```python
from build123d import *

# Parameters (mm, degrees)
F0_W      = 149
F0_H      = 43
F1_DEPTH  = 7
F2_T      = -1.6
F3_DEPTH  = 1
F4_W      = 1.6
F4_H      = 5
F5_DEPTH  = 6.6
F6_W      = 5
F6_H      = 1.0360542744
F7_DEPTH  = 1
F8_SIZE   = 1
F9_W      = 5
F9_H      = 1.0135311693
F10_DEPTH = 1
F11_SIZE  = 1
F12_W     = 6.7361369729
F12_H     = 9.1
F13_DEPTH = 25


with BuildPart() as f1:
    # F0 (on Top) → F1 (new body)
    with BuildSketch(Plane.XY):
        with Locations((74.5, -21.5)):
            Rectangle(F0_W, F0_H)
    extrude(amount=F1_DEPTH)

    # F2
    f2_openings = [f1.faces().sort_by_distance(p)[0] for p in [
        (74.5, -21.5, 7),
    ]]
    offset(amount=F2_T, openings=f2_openings)

    # F3 (add): a face of the model
    f3_faces = [f1.faces().sort_by_distance(p)[0] for p in [
        (74.5, -21.5, 1.6),
    ]]
    extrude(f3_faces, amount=F3_DEPTH)

    # F4 (on face) → F5 (join)
    with BuildSketch(Plane.XY.offset(7)):
        with Locations((0.8, -6.7)):
            Rectangle(F4_W, F4_H)
        with Locations((0.8, -36.3)):
            Rectangle(F4_W, F4_H)
        with Locations((148.2, -6.7)):
            Rectangle(F4_W, F4_H)
        with Locations((148.2, -36.3)):
            Rectangle(F4_W, F4_H)
    extrude(amount=F5_DEPTH)

    # F6 (on face) → F7 (join)
    with BuildSketch(Plane(origin=(0, 0, 0), x_dir=(0, -1, 0), z_dir=(-1, 0, 0))):
        with Locations((6.7, 13.0819728628)):
            Rectangle(F6_W, F6_H)
        with Locations((36.3, 13.0819728628)):
            Rectangle(F6_W, F6_H)
    extrude(amount=F7_DEPTH)

    # F8
    f8_edges = [f1.edges().sort_by_distance(p)[0] for p in [
        (-1, -6.7, 13.6),
        (-1, -36.3, 13.6),
    ]]
    chamfer(f8_edges, length=F8_SIZE)

    # F9 (on face) → F10 (join)
    with BuildSketch(Plane.YZ.offset(149)):
        with Locations((-36.3, 13.0932344154)):
            Rectangle(F9_W, F9_H)
        with Locations((-6.7, 13.0932344154)):
            Rectangle(F9_W, F9_H)
    extrude(amount=F10_DEPTH)

    # F11
    f11_edges = [f1.edges().sort_by_distance(p)[0] for p in [
        (150, -36.3, 13.6),
        (150, -6.7, 13.6),
    ]]
    chamfer(f11_edges, length=F11_SIZE)

    # F12 (on face) → F13 (cut)
    with BuildSketch(Plane(origin=(0, 0, 0), x_dir=(1, 0, 0), z_dir=(0, 0, -1))):
        with Locations((77.8680684865, 26.05)):
            Rectangle(F12_W, F12_H)
        with Locations((71.1319315135, 26.05)):
            Rectangle(F12_W, F12_H)
        with Locations((77.8680684865, 16.95)):
            Rectangle(F12_W, F12_H)
        with Locations((71.1319315135, 16.95)):
            Rectangle(F12_W, F12_H)
    extrude(amount=-F13_DEPTH, mode=Mode.SUBTRACT)


solid = f1.part
```
CAD build for the part. Positions are in the model's coordinates, mm. A direction names the side the tool comes from. Round coordinates to 2 decimals unless told otherwise and drop trailing zeros. Write each loop counter-clockwise with the first axis right and the second up, starting at its lowest first coordinate (ties: lowest second). Pieces come first, ordered by that corner, then holes. Notation, with made-up numbers: M -27,-15.75 L 6,-15.75 A13 ccw 6,-7.75 Z; hole C -14,74 d10. An arc over 180 degrees is marked long. One line per question, with ' | ' between items.
1. Cut at C-C on y = -18. Write the cut outline in (x, z).
Working result:
outline: M 0,0 L 67.76,0 L 67.76,2.6 L 1.6,2.6 L 1.6,7 L 0,7 Z; M 81.24,0 L 149,0 L 149,7 L 147.4,7 L 147.4,2.6 L 81.24,2.6 Z
2. Probe L1, parallel to X at y = -30.5, z = 4; L2, parallel to Y at x = 45, z = 4.5; L3, parallel to X at y = -15, z = 2.5. List the from-to ranges inside material, lowest first. Write a range as from..to.
Working result:
L1: 0..1.6, 147.4..149 | L2: -43..-41.4, -1.6..0 | L3: 0..67.76, 81.24..149
3. Which spindle directions (+Z, -Z, +X, -X, +Y, -Y) get a long thin tool onto all of the face, cutting with end or side? Do faces 1 (the flat face through (73, -1.6, 5)), 2 (the flat face through (1, -4.2, 10)), 3 (the flat face through (74, -12.4, 1)). Say none if no direction does.
Working result:
face 1: +Z | face 2: +Z, +X, -X, +Y | face 3: +Z, -Z
4. Cut at A-A on x = 69.5. Write the cut outline in (y, z), and give its area (3 significant figures).
Working result:
outline: M -43,0 L -30.6,0 L -30.6,2.6 L -41.4,2.6 L -41.4,7 L -43,7 Z; M -12.4,0 L 0,0 L 0,7 L -1.6,7 L -1.6,2.6 L -12.4,2.6 Z | area: 78.6 mm2
5. Cut at B-B on z = 5.25. Write the cut outline in (x, y).
Working result:
outline: M 0,-43 L 149,-43 L 149,0 L 0,0 Z; hole M 1.6,-41.4 L 147.4,-41.4 L 147.4,-1.6 L 1.6,-1.6 Z
6. Pin check, flat tips, straight feed: pin 1 Ø1.8 at (x, y) = (0.5, -18) entering from +Z; pin 2 Ø3.5 at (y, z) = (-13.5, 5.5) entering from +X; pin 3 Ø1.3 at (x, z) = (149, 9) entering from +Y; pin 4 Ø1 at (x, z) = (118, 9) entering from +Y. Stop position of each tip, or through.
Working result:
pin 1: z = 7 | pin 2: x = 149 | pin 3: y = -4.2 | pin 4: through
7. Mould opens along Y. For faces 4 (the flat face through (81.236, -21, 1)), 5 (the flat face through (73, 0, 3)), 6 (the flat face through (1, -38.8, 10)) say: pulls with the +Y half, pulls with the -Y half, needs draft (parallel to the pull), parting line crosses it, or undercut.
Working result:
face 4: undercut | face 5: pulls with the +Y half | face 6: pulls with the -Y half
